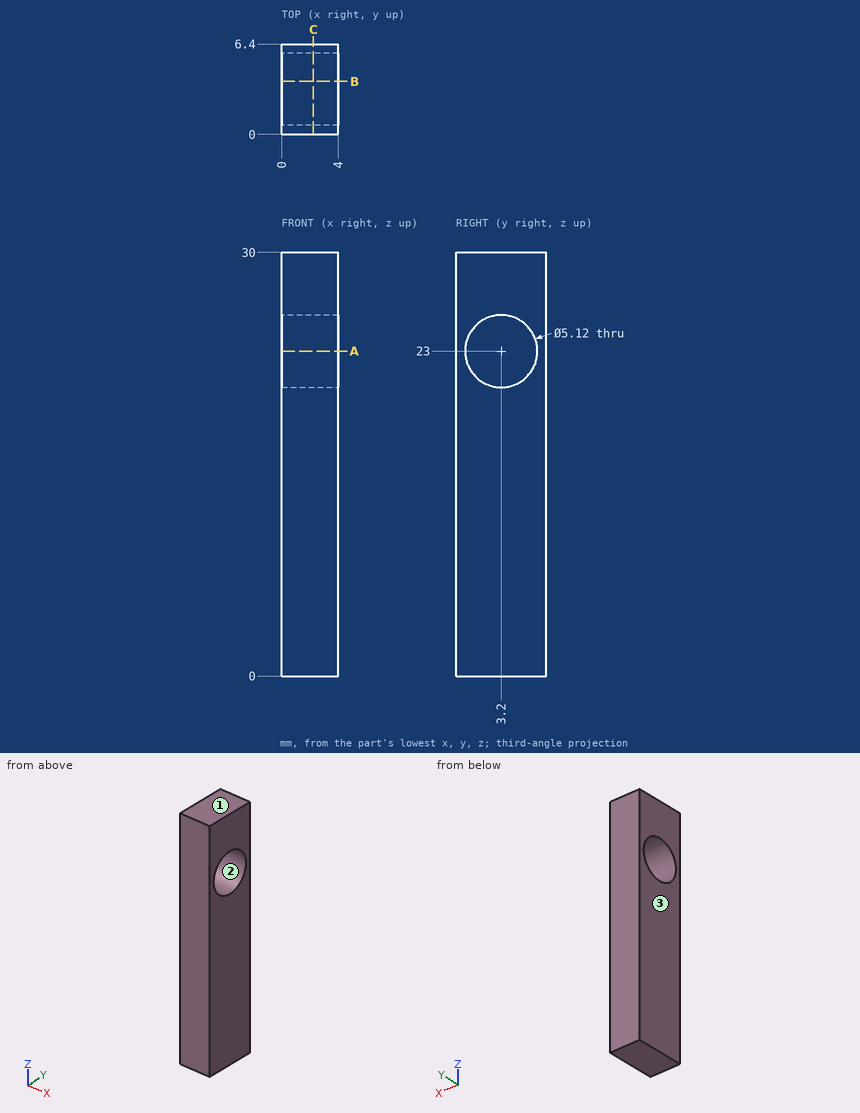
Verification items for this drawing (mm, ordinates from the low corner). Give positions to 0.01 mm unless a question says otherwise; leave off trailing zeros. Order: outer loops, then holes, each group sorted by start corner. A loop starts at its lowest first (then second) coordinate and runs counter-clockwise, first axis right, second up. Notation, with made-up numbers: M 4,16 L 49,16 A14 cw 49,31 Z; hole C -35.75,54.25 d10. An arc over 180 degrees is marked long. Use a Markdown table: item, result.
Item 1: Draft check along Z on the marked faces 1, 2 and 3. Enter one of: +Z half, -Z half, draft (parallel to the pull), parting line (faces both ways), or undercut.
Answers follow:
| item | result |
|---|---|
| face 1 | +Z half |
| face 2 | undercut |
| face 3 | draft |
Item 2: Material ranges on line 1 along Y through (x, z) = (2.55, 23); line 2 along Z through (x, y) = (2.8, 3.25); line 3 along Y through (x, z) = (1.7, 21.5), recorded low to high.
Answers follow:
| item | result |
|---|---|
| line 1 | y = 0 to 0.64, 5.76 to 6.4 |
| line 2 | z = 0 to 20.44, 25.56 to 30 |
| line 3 | y = 0 to 1.13, 5.27 to 6.4 |
Item 3: Section check C-C (x = 2.25). Record the cut outline in (y, z).
Answers follow:
| item | result |
|---|---|
| outline | M 0,0 L 6.4,0 L 6.4,30 L 0,30 Z; hole C 3.2,23 d5.12 |
Item 4: Section check B-B (y = 3.75). Record the cut outline in (x, z), and give its area (4 significant figures).
Answers follow:
| item | result |
|---|---|
| outline | M 0,0 L 4,0 L 4,20.5 L 0,20.5 Z; M 0,25.5 L 4,25.5 L 4,30 L 0,30 Z |
| area | 100.0 mm2 |
Item 5: Section check A-A (z = 23). Record the cut outline in (x, y).
Answers follow:
| item | result |
|---|---|
| outline | M 0,0 L 4,0 L 4,0.64 L 0,0.64 Z; M 0,5.76 L 4,5.76 L 4,6.4 L 0,6.4 Z |
